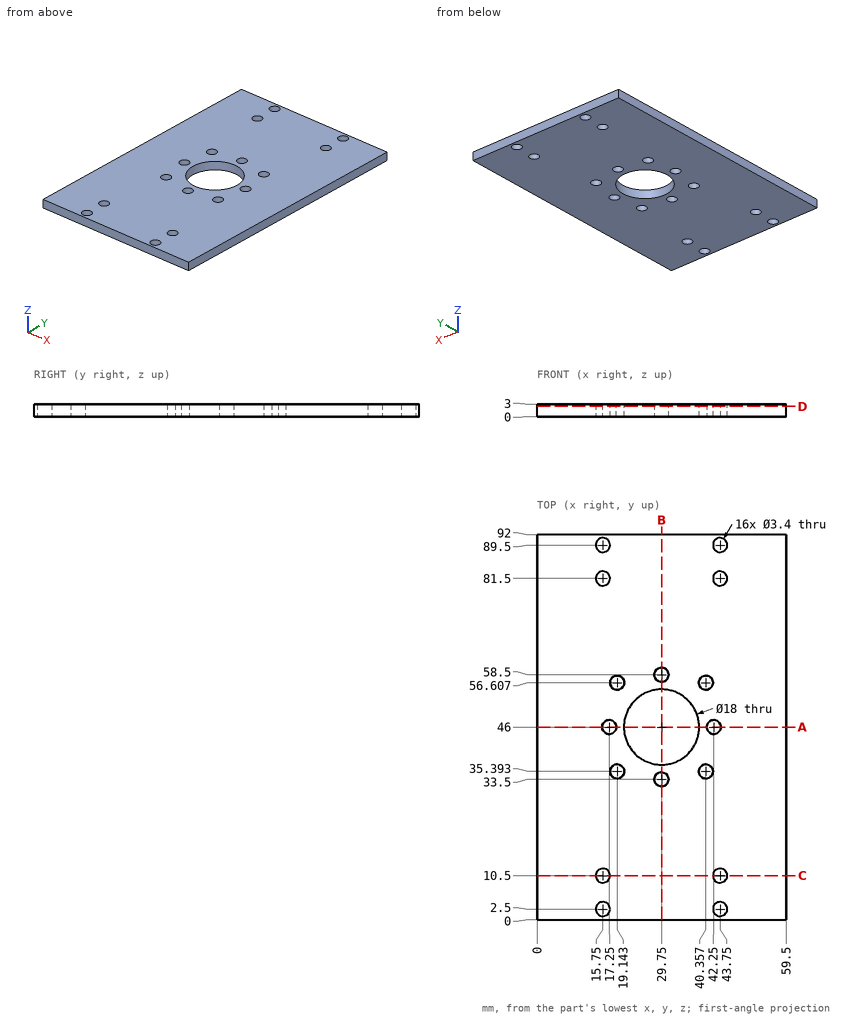
Print and shaded views of the part. All mm, measured from the part's lowest x, y and z. Give positions to 0.01 mm unless a question says otherwise; leave off trailing zeros. Loops run counter-clockwise (first coordinate to the right, second up) from the corner with the lowest first, then second, coordinate; pieces in that order, holes last. Notation, with made-up numbers: (4.5, -37.5) -> (11.5, -37.5) arc R21 ccw to (11.5, -8.5) -> close; hole circle Ø5 at (43, 86). An arc over 180 degrees is marked (long way). Use a Markdown table: item, result.
1. Slice it at B-B (x = 29.75). List the corners of the cut face in (y, z).
Check result:
| item | result |
|---|---|
| outline | (0, 0) -> (31.8, 0) -> (31.8, 3) -> (0, 3) -> close; (35.2, 0) -> (37, 0) -> (37, 3) -> (35.2, 3) -> close; (55, 0) -> (56.8, 0) -> (56.8, 3) -> (55, 3) -> close; (60.2, 0) -> (92, 0) -> (92, 3) -> (60.2, 3) -> close |
2. Wall check: L1, parallel to X at y = 81.5, z = 2.3; L2, parallel to Y at x = 44, z = 2.45; L3, parallel to Y at x = 29.75, z = 1.45. Give the ranges that are in metal, low to high. Write a range as [from, to].
Check result:
| item | result |
|---|---|
| L1 | x = [0, 14.05], [17.45, 42.05], [45.45, 59.5] |
| L2 | y = [0, 0.82], [4.18, 8.82], [12.18, 79.82], [83.18, 87.82], [91.18, 92] |
| L3 | y = [0, 31.8], [35.2, 37], [55, 56.8], [60.2, 92] |
3. Slice it at C-C (y = 10.5). List the corners of the cut face in (x, z), plus the area to 3 significant figures.
Check result:
| item | result |
|---|---|
| outline | (0, 0) -> (14.05, 0) -> (14.05, 3) -> (0, 3) -> close; (17.45, 0) -> (42.05, 0) -> (42.05, 3) -> (17.45, 3) -> close; (45.45, 0) -> (59.5, 0) -> (59.5, 3) -> (45.45, 3) -> close |
| area | 158 mm^2 |
4. Slice it at D-D (z = 2.45). Give the number of separate pieces and of enclosed holes in the cut face, plus the area to 3 significant figures.
Check result:
| item | result |
|---|---|
| separate pieces | 1 |
| enclosed holes | 17 |
| area | 5,070 mm^2 |
5. Slice it at A-A (y = 46). List the corners of the cut face in (x, z), plus the area to 3 significant figures.
Check result:
| item | result |
|---|---|
| outline | (0, 0) -> (15.55, 0) -> (15.55, 3) -> (0, 3) -> close; (18.95, 0) -> (20.75, 0) -> (20.75, 3) -> (18.95, 3) -> close; (38.75, 0) -> (40.55, 0) -> (40.55, 3) -> (38.75, 3) -> close; (43.95, 0) -> (59.5, 0) -> (59.5, 3) -> (43.95, 3) -> close |
| area | 104 mm^2 |
